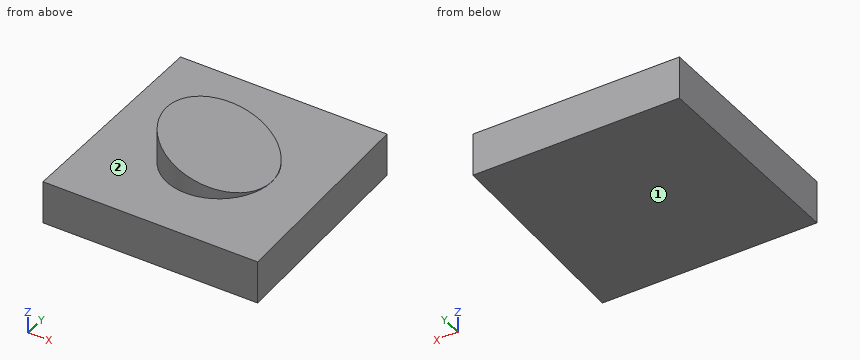
```python
from build123d import *

# Parameters (mm, degrees)
F1_DEPTH = 28.702
F2_R     = 35.250577
F3_DEPTH = 25.4
F5_DEPTH = 144.567961


with BuildPart() as f1:
    # F0 (on Top) → F1 (new body)
    with BuildSketch(Plane.XY):
        Polygon((65.11163, 74.948795), (-74.116208, 74.948795), (-74.116208, -69.618165), (70.669487, -69.618165), align=None)
    extrude(amount=F1_DEPTH)

    # F2 (on face) → F3 (join)
    with BuildSketch(Plane.XY.offset(28.702)):
        Circle(F2_R)
    extrude(amount=F3_DEPTH)

    # F4 (on face) → F5 (cut, through all)
    with BuildSketch(Plane.XZ.offset(69.618165)):
        Polygon((35.616178, 54.999514), (-38.837059, 55.3034), (35.616178, 28.702), align=None)
    extrude(amount=-F5_DEPTH, mode=Mode.SUBTRACT)


solid = f1.part
```
Input: part model. Units: mm. Frame: model coordinates. Face numbers are marked on the shaded views. A direction names the side the tool comes from. Give positions to 0.01 mm unless a question says otherwise; leave off trailing zeros. Order: outer loops, then holes, each group sorted by start corner. A loop starts at its lowest first (then second) coordinate and runs counter-clockwise, first axis right, second up. Notation, with made-up numbers: (-21.5, 45.25) - (13.5, 45.25) arc R18 ccw to (13.5, 79.25) - close; hole circle Ø2 at (82, 51). An arc over 180 degrees is marked (long way). Use a Markdown table: item, result.
(1) Pin query (flat end, axial travel): pin 1 (10 mm diameter, centred on x = 29, z = 41.5, fed in from +Y); pin 2 (4 mm diameter, centred on x = -7, y = 58.5, fed in from +Z); pin 3 (4 mm diameter, centred on x = -8.5, z = 42, fed in from +Y); pin 4 (3 mm diameter, centred on y = -11, z = 15.5, fed in from +X). Return the tip coordinate at first contact, or that it passes through.
Computed values:
| item | result |
|---|---|
| pin 1 | passes through |
| pin 2 | stops at z = 28.7 |
| pin 3 | stops at y = 34.65 |
| pin 4 | stops at x = 68.47 |
(2) Section query C-C (z = 8). Output: boundary loops of the cut face in (x, y), then the cut area to 3 significant figures.
Computed values:
| item | result |
|---|---|
| outline | (-74.12, -69.62) - (70.67, -69.62) - (65.11, 74.95) - (-74.12, 74.95) - close |
| area | 20,500 mm2 |
(3) Section query A-A (y = 23). Output: boundary loops of the cut face in (x, z).
Computed values:
| item | result |
|---|---|
| outline | (-74.12, 0) - (67.11, 0) - (67.11, 28.7) - (26.71, 28.7) - (26.71, 31.88) - (-26.71, 50.97) - (-26.71, 28.7) - (-74.12, 28.7) - close |
(4) Section query B-B (x = 0). Output: boundary loops of the cut face in (y, z), then the cut area to 3 significant figures.
Computed values:
| item | result |
|---|---|
| outline | (-69.62, 0) - (74.95, 0) - (74.95, 28.7) - (35.25, 28.7) - (35.25, 41.43) - (-35.25, 41.43) - (-35.25, 28.7) - (-69.62, 28.7) - close |
| area | 5,050 mm2 |
(5) Line query: line 1 (Z direction, x = 34.5, y = -57); line 2 (X direction, y = -60, z = 25); line 3 (Z direction, x = 26, y = 3). Output: solid intervals per line, ascending. Write a range as from..to.
Computed values:
| item | result |
|---|---|
| line 1 | z = 0..28.7 |
| line 2 | x = -74.12..70.3 |
| line 3 | z = 0..32.14 |
(6) Section query D-D (y = -52.5). Output: boundary loops of the cut face in (x, z).
Computed values:
| item | result |
|---|---|
| outline | (-74.12, 0) - (70.01, 0) - (70.01, 28.7) - (-74.12, 28.7) - close |
(7) Access query for the marked faces 1 and 2. Directions: +Z, -Z, +X, -X, +Y, -Y. A direction counts if a zero-diameter tool reaches every point of the face in a straight line with its end or side. Return the directions, or none.
Computed values:
| item | result |
|---|---|
| face 1 | -Z, +X, -X, +Y, -Y |
| face 2 | +Z |
